from build123d import *

# Parameters (mm, degrees)
SKETCH1_W           = 48
SKETCH1_H           = 20
BOSS_EXTRUDE1_DEPTH = 10
SKETCH4_W           = 48
SKETCH4_H           = 5.8
BOSS_EXTRUDE2_DEPTH = 1
SKETCH2_R           = 2.6
CUT_EXTRUDE1_DEPTH  = 12


with BuildPart() as part:
    # Sketch1 → Boss-Extrude1 (new body)
    with BuildSketch(Plane.XY):
        Rectangle(SKETCH1_W, SKETCH1_H)
    extrude(amount=BOSS_EXTRUDE1_DEPTH)

    # Sketch4 → Boss-Extrude2 (add)
    with BuildSketch(Plane.XY.offset(10)):
        Rectangle(SKETCH4_W, SKETCH4_H)
    extrude(amount=BOSS_EXTRUDE2_DEPTH)

    # Sketch2 → Cut-Extrude1 (cut, through all)
    with BuildSketch(Plane.XY):
        with Locations((-15.95, 0)):
            Circle(SKETCH2_R)
    cut_extrude1 = extrude(amount=CUT_EXTRUDE1_DEPTH, mode=Mode.SUBTRACT)

    # Mirror1: Cut-Extrude1 across plane
    add(cut_extrude1.mirror(Plane(origin=(0, 0, 0), x_dir=(0, 0, 1), z_dir=(1, 0, 0))), mode=Mode.SUBTRACT)


solid = part.part
Geometry: final body of the model. Coordinates: model frame, mm. A direction names the side the tool comes from. Round coordinates to 2 decimals unless told otherwise and drop trailing zeros. Order: outer loops, then holes, each group sorted by start corner. A loop starts at its lowest first (then second) coordinate and runs counter-clockwise, first axis right, second up.
Q1. Section D-D, the plane z = 2.75. Output: boundary loops of the cut face in (x, y), and give its area (3 significant figures).
Result sheet:
outline: (-24, -10) - (24, -10) - (24, 10) - (-24, 10) - close; hole circle Ø5.2 at (-15.95, 0); hole circle Ø5.2 at (15.95, 0)
area: 918 mm2
Q2. Mould query, pull axis Y, two halves, no side actions, for faces 4 (the face through (-18.547, 0.114, 5.423)), 5 (the face through (0, -6, 10)), 6 (the face through (18.547, 0.114, 5.423)), 7 (the face through (-0.3, 2.9, 10.5)). Classes: released by +Y, released by -Y, zero draft, split by the parting line, or undercut.
Result sheet:
face 4: undercut
face 5: zero draft
face 6: undercut
face 7: released by +Y
Q3. Material intervals for probe 1 along Y at (x, z) = (-15.95, 3); probe 2 along X at (y, z) = (1.25, 3.5); probe 3 along Z at (x, y) = (5, 8.25), sorted ascending.
Result sheet:
probe 1: y = -10 to -2.6, 2.6 to 10
probe 2: x = -24 to -18.23, -13.67 to 13.67, 18.23 to 24
probe 3: z = 0 to 10
Q4. Pin query (flat end, axial travel): pin 1 (0.8 mm diameter, centred on x = 7, z = 10.5, fed in from +Y); pin 2 (2 mm diameter, centred on x = -4, y = 5.5, fed in from +Z); pin 3 (4 mm diameter, centred on x = -15.95, y = 0, fed in from +Z). Return the tip coordinate at first contact, or that it passes through.
Result sheet:
pin 1: stops at y = 2.9
pin 2: stops at z = 10
pin 3: passes through
Q5. Section A-A, the plane y = 0. Output: boundary loops of the cut face in (x, z).
Result sheet:
outline: (-24, 0) - (-18.55, 0) - (-18.55, 11) - (-24, 11) - close; (-13.35, 0) - (13.35, 0) - (13.35, 11) - (-13.35, 11) - close; (18.55, 0) - (24, 0) - (24, 11) - (18.55, 11) - close
Q6. Section C-C, the plane x = -8.5. Output: boundary loops of the cut face in (y, z), and give its area (3 significant figures).
Result sheet:
outline: (-10, 0) - (10, 0) - (10, 10) - (2.9, 10) - (2.9, 11) - (-2.9, 11) - (-2.9, 10) - (-10, 10) - close
area: 206 mm2
Q7. Access query for faces 1 (the face through (0, 6, 10)), 2 (the face through (0, 0, 0)), 3 (the face through (-0.3, -2.9, 10.5)). Directions: +Z, -Z, +X, -X, +Y, -Y. A direction counts if a zero-diameter tool reaches every point of the face in a straight line with its end or side. Return the directions, or none.
Result sheet:
face 1: +Z, +X, -X, +Y
face 2: -Z, +X, -X, +Y, -Y
face 3: +Z, +X, -X, -Y
Q8. Section B-B, the plane x = -15.95. Output: boundary loops of the cut face in (y, z), and give its area (3 significant figures).
Result sheet:
outline: (-10, 0) - (-2.6, 0) - (-2.6, 11) - (-2.9, 11) - (-2.9, 10) - (-10, 10) - close; (2.6, 0) - (10, 0) - (10, 10) - (2.9, 10) - (2.9, 11) - (2.6, 11) - close
area: 149 mm2
